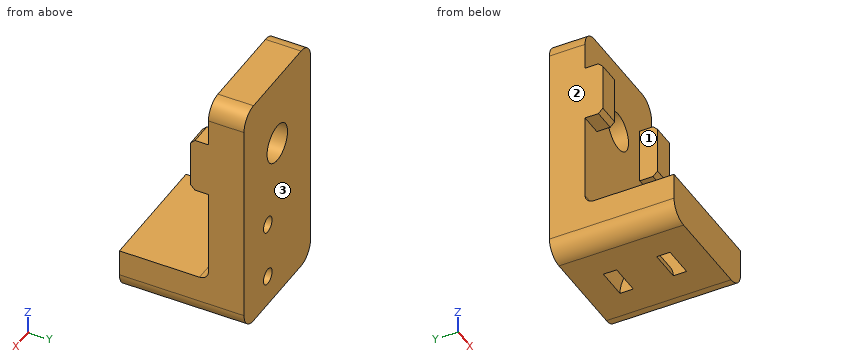
```python
from build123d import *

# Parameters (mm, degrees)
SKETCH2_W           = 14
SKETCH2_H           = 22
SKETCH2_H_2         = 5
BOSS_EXTRUDE1_DEPTH = 4
SKETCH4_W           = 14
SKETCH4_H           = 6.25
BOSS_EXTRUDE2_DEPTH = 2
SKETCH3_R           = 0.9
SKETCH3_R_2         = 2.15
CUT_EXTRUDE1_DEPTH  = 27.758176321
CHAMFER1_SIZE       = 0.5
FILLET1_R           = 2
CUT_EXTRUDE2_REACH  = 28.758
SKETCH5_W           = 9
SKETCH5_H           = 6.25
BOSS_EXTRUDE3_DEPTH = 10
SKETCH7_W           = 3.5
SKETCH7_H           = 1.5
FILLET2_R           = 1


with BuildPart() as part:
    # Sketch2 → Boss-Extrude1 (new body)
    with BuildSketch(Plane(origin=(0, 0, 0), x_dir=(1, 0, 0), z_dir=(0, 1, 0))):
        with Locations((7, 11)):
            Rectangle(SKETCH2_W, SKETCH2_H)
        with Locations((7, -2.5)):
            Rectangle(SKETCH2_W, SKETCH2_H_2)
    extrude(amount=BOSS_EXTRUDE1_DEPTH)

    # Sketch4 → Boss-Extrude2 (add)
    with BuildSketch(Plane(origin=(0, 0, 0), x_dir=(-1, 0, 0), z_dir=(0, -1, 0))):
        with Locations((-7, 3.125)):
            Rectangle(SKETCH4_W, SKETCH4_H)
    extrude(amount=BOSS_EXTRUDE2_DEPTH)

    # Sketch3 → Cut-Extrude1 (cut, through all)
    with BuildSketch(Plane(origin=(0, 4, 0), x_dir=(1, 0, 0), z_dir=(0, 1, 0))):
        with Locations(Location((9, 18.5, 0), (0, 0, 180))):
            Circle(SKETCH3_R)
        with Locations(Location((9, 12, 0), (0, 0, 180))):
            Circle(SKETCH3_R)
        with Locations(Location((7, 3.125, 0), (0, 0, 180))):
            Circle(SKETCH3_R_2)
    extrude(amount=-CUT_EXTRUDE1_DEPTH, mode=Mode.SUBTRACT)

    # Chamfer1
    chamfer1_edges = [part.edges().sort_by_distance(p)[0] for p in [
        (7, -2, -6.25),
        (7, -2, 0),
    ]]
    chamfer(chamfer1_edges, length=CHAMFER1_SIZE)

    # Fillet1
    fillet1_edges = [part.edges().sort_by_distance(p)[0] for p in [
        (0, 2, -22),
        (14, 2, -22),
        (14, 2, 5),
        (0, 2, 5),
    ]]
    fillet(fillet1_edges, radius=FILLET1_R)

    # Cut-Extrude2: up to this face of the body (flat: up to its plane)
    cut_extrude2_end = Plane(part.part.faces().sort_by_distance((6.952367547, 0, -14.038528118))[0])
    # Sketch5 → Cut-Extrude2 (cut, up to the picked face)
    with BuildSketch(Plane.XZ.offset(2), mode=Mode.PRIVATE) as cut_extrude2_sk1:
        with Locations((7, -3.125)):
            Rectangle(SKETCH5_W, SKETCH5_H)
    cut_extrude2_tool1 = split(extrude(cut_extrude2_sk1.sketch, amount=-CUT_EXTRUDE2_REACH, mode=Mode.PRIVATE), bisect_by=cut_extrude2_end, keep=Keep.BOTH, mode=Mode.PRIVATE)
    add(cut_extrude2_tool1.solids().sort_by(Axis((7, -2, -3.125), (0, 1, 0)))[0], mode=Mode.SUBTRACT)

    # Sketch6 → Boss-Extrude3 (add)
    with BuildSketch(Plane.XZ):
        with BuildLine():
            Line((0, -17), (0, -20))
            ThreePointArc((0, -20), (0.585786438, -21.414213562), (2, -22))
            Line((2, -22), (12, -22))
            ThreePointArc((12, -22), (13.414213562, -21.414213562), (14, -20))
            Line((14, -20), (14, -17))
            Line((14, -17), (0, -17))
        make_face()
    extrude(amount=BOSS_EXTRUDE3_DEPTH)

    # Sketch7 → Cut-Revolve1 (revolve, cut)
    with BuildSketch(Plane(origin=(0, 0, -22), x_dir=(-1, 0, 0), z_dir=(0, 0, -1))):
        with Locations((-7, 0)):
            Rectangle(SKETCH7_W, SKETCH7_H)
    revolve(axis=Axis((14, -3, -22), (-1, 0, 0)), mode=Mode.SUBTRACT)

    # Fillet2
    fillet2_edges = [part.edges().sort_by_distance(p)[0] for p in [
        (7, 0, -17),
    ]]
    fillet(fillet2_edges, radius=FILLET2_R)


solid = part.part
```
Check sheet for the modelled part. Datum: model origin and axes. Units: mm. Face numbers are marked on the shaded views. Give positions to 0.01 mm unless a question says otherwise; leave off trailing zeros. Write each loop counter-clockwise with the first axis right and the second up, starting at its lowest first coordinate (ties: lowest second). Pieces come first, ordered by that corner, then holes. Notation, with made-up numbers: (28, 85) -> (74, 85) arc R22 ccw to (74, 103) -> close; hole circle Ø6 at (76.25, 6). An arc over 180 degrees is marked (long way). Use CSV: the item, a comma, the result in double quotes. Start each with the question number.
Q1. Cross-section at D-D on y = -3.75. Enter the section's corners in (x, z).
Q2. Cross-section at B-B on y = 2.75. Enter the section's corners in (x, z) (3 decimals).
Q3. Cross-section at C-C on x = 3. Enter the section's corners in (y, z).
Q4. Depth check by flat-ended pin: P1, Ø4, axis at x = 10.5, z = -6, coming from the -Y side; P2, Ø1.2, axis at x = 13, y = -0.5, coming from the +Z side (3 decimals); P3, Ø0.8, axis at x = 1, y = -1, coming from the -Z side. Enter the tip coordinate at first touch or a pass-through.
Q5. Cross-section at A-A on z = -12. Enter the section's corners in (x, y).
Q6. Release check for a two-part mould opening along X. For the marked faces 1, 2 and 3 record: +X half, -X half, draft (parallel to the pull), parting line (faces both ways), or undercut.
Q7. Scan lines: line 1 along X through (y, z) = (-4.5, -19); line 2 along Z through (x, y) = (7, 3.15) (3 decimals); line 3 along Y through (x, z) = (1.75, -3). Record each from-to range of solid material in increasing order.
Working result:
1,outline,"(0, -20) arc R2 ccw to (2, -22) -> (12, -22) arc R2 ccw to (14, -20) -> (14, -17) -> (0, -17) -> close; hole (5.25, -19.88) -> (8.75, -19.88) -> (8.75, -18.33) -> (5.25, -18.33) -> close"
2,outline,"(0, -20) arc R2 ccw to (2, -22) -> (12, -22) arc R2 ccw to (14, -20) -> (14, 3) arc R2 ccw to (12, 5) -> (2, 5) arc R2 ccw to (0, 3) -> close; hole circle Ø4.3 at (7, -3.125); hole circle Ø1.8 at (9, -18.5); hole circle Ø1.8 at (9, -12)"
3,outline,"(-10, -22) -> (4, -22) -> (4, 5) -> (0, 5) -> (0, -16) arc R1 cw to (-1, -17) -> (-10, -17) -> close"
4,P1,"stops at y = -2"
4,P2,"stops at z = 4.885"
4,P3,"stops at z = -21.91"
5,outline,"(0, 0) -> (8.1, 0) -> (8.1, 4) -> (0, 4) -> close; (9.9, 0) -> (14, 0) -> (14, 4) -> (9.9, 4) -> close"
6,face 1,"undercut"
6,face 2,"-X half"
6,face 3,"draft"
7,line 1,"x = 0 to 5.25, 8.75 to 14"
7,line 2,"z = -22 to -5.275, -0.975 to 5"
7,line 3,"y = -2 to 4"
